from build123d import *

# Parameters (mm, degrees)
SKETCH_1_W          = 10
SKETCH_1_H          = 10
SKETCH_1_W_2        = 8
SKETCH_1_H_2        = 8
EXTRUDE_2_DEPTH     = 80
SKETCH_2_R          = 2
CUT_EXTRUDE_1_DEPTH = 70
SKETCH_3_R          = 2
CUT_EXTRUDE_2_DEPTH = 104
SKETCH_4_R          = 2
CUT_EXTRUDE_3_DEPTH = 104
SKETCH_5_R          = 2
CUT_EXTRUDE_4_DEPTH = 100
SKETCH_6_R          = 2
CUT_EXTRUDE_5_DEPTH = 10


with BuildPart() as part:
    # 草图1 → 凸台-拉伸2 (new body)
    with BuildSketch(Plane.XY):
        with Locations((5, 5)):
            Rectangle(SKETCH_1_W, SKETCH_1_H)
        with Locations((5, 5)):
            Rectangle(SKETCH_1_W_2, SKETCH_1_H_2, mode=Mode.SUBTRACT)
    extrude(amount=EXTRUDE_2_DEPTH)

    # 草图2 → 切除-拉伸1 (cut)
    with BuildSketch(Plane(origin=(0, 10, 0), x_dir=(1, 0, 0), z_dir=(0, 1, 0))):
        with Locations(Location((5, -72, 0), (0, 0, 180))):
            Circle(SKETCH_2_R)
        with Locations(Location((5, -8, 0), (0, 0, 180))):
            Circle(SKETCH_2_R)
    extrude(amount=-CUT_EXTRUDE_1_DEPTH, mode=Mode.SUBTRACT)

    # 草图3 → 切除-拉伸2 (cut)
    with BuildSketch(Plane.XZ):
        with Locations((5, 25)):
            Circle(SKETCH_3_R)
    extrude(amount=-CUT_EXTRUDE_2_DEPTH, mode=Mode.SUBTRACT)

    # 草图4 → 切除-拉伸3 (cut)
    with BuildSketch(Plane.XZ):
        with Locations((5, 55)):
            Circle(SKETCH_4_R)
    extrude(amount=-CUT_EXTRUDE_3_DEPTH, mode=Mode.SUBTRACT)

    # 草图5 → 切除-拉伸4 (cut)
    with BuildSketch(Plane(origin=(10, 0, 0), x_dir=(0, 0, -1), z_dir=(1, 0, 0))):
        with Locations(Location((-16, 5, 0), (0, 0, 90))):
            Circle(SKETCH_5_R)
    extrude(amount=-CUT_EXTRUDE_4_DEPTH, mode=Mode.SUBTRACT)

    # 草图6 → 切除-拉伸5 (cut)
    with BuildSketch(Plane.ZY):
        with Locations(Location((55, 5, 0), (0, 0, 270))):
            Circle(SKETCH_6_R)
    extrude(amount=-CUT_EXTRUDE_5_DEPTH, mode=Mode.SUBTRACT)


solid = part.part
CAD build for the part. Positions are in the model's coordinates, mm. A direction names the side the tool comes from. Give positions to 0.01 mm unless a question says otherwise; leave off trailing zeros. Write each loop counter-clockwise with the first axis right and the second up, starting at its lowest first coordinate (ties: lowest second). Pieces come first, ordered by that corner, then holes. Notation, with made-up numbers: (0, 19) - (41, 19) arc R21 ccw to (41, 31) - close; hole circle Ø6 at (-2.75, 41). An arc over 180 degrees is marked (long way). Put each result on its own line as item: value.
(1) Saw through at C-C (z = 51). List the corners of the cut face in (x, y).
Working result:
outline: (0, 0) - (10, 0) - (10, 10) - (0, 10) - close; hole (1, 1) - (9, 1) - (9, 9) - (1, 9) - close
(2) Saw through at B-B (y = 5). List the corners of the cut face in (x, z), then the cut area to 3 significant figures.
Working result:
outline: (0, 0) - (1, 0) - (1, 14) - (0, 14) - close; (0, 18) - (1, 18) - (1, 53) - (0, 53) - close; (0, 57) - (1, 57) - (1, 80) - (0, 80) - close; (9, 0) - (10, 0) - (10, 14) - (9, 14) - close; (9, 18) - (10, 18) - (10, 53) - (9, 53) - close; (9, 57) - (10, 57) - (10, 80) - (9, 80) - close
area: 144 mm^2
(3) Drop a flat-ended pin along its axis: pin 1 Ø3.5 at (x, z) = (5, 72) entering from +Y. Give the stop position or say it passes through.
Working result:
pin 1: through
(4) Saw through at D-D (z = 24). List the corners of the cut face in (x, y).
Working result:
outline: (0, 0) - (3.27, 0) - (3.27, 1) - (1, 1) - (1, 9) - (3.27, 9) - (3.27, 10) - (0, 10) - close; (6.73, 0) - (10, 0) - (10, 10) - (6.73, 10) - (6.73, 9) - (9, 9) - (9, 1) - (6.73, 1) - close
(5) Pull direction X, two halves, no side cores. Call faces 3 (the flat face through (10, 5, 39)), 4 (the flat face through (5, 0, 39)), 5 (the flat face through (9, 5, 39)): released by +X, released by -X, zero draft, split by the parting line, or undercut.
Working result:
face 3: released by +X
face 4: zero draft
face 5: undercut
(6) Saw through at A-A (x = 7.75). List the corners of the cut face in (y, z).
Working result:
outline: (0, 0) - (1, 0) - (1, 80) - (0, 80) - close; (9, 0) - (10, 0) - (10, 80) - (9, 80) - close
(7) Wall check: L1, parallel to Y at x = 8, z = 66; L2, parallel to Z at x = 5, y = 0.45. Give the ranges that are in metal, low to high.
Working result:
L1: 0 to 1, 9 to 10
L2: 0 to 6, 10 to 23, 27 to 53, 57 to 70, 74 to 80
(8) Tool access for faces 1 (the cylindrical face through (9.493, 5.26, 56.983)), 2 (the flat face through (5, 9, 39)): list every direction of +Z, -Z, +X, -X, +Y, -Y with a clear straight run to the whole face (end or side of a thin tool).
Working result:
face 1: +X, -X
face 2: +Z, -Z
